Job drawing, mm, ordinate dimensions from the low corner. One solid piece. A direction names the side the tool comes from. Give positions to 0.01 mm unless a question says otherwise; leave off trailing zeros. Order: outer loops, then holes, each group sorted by start corner. A loop starts at its lowest first (then second) coordinate and runs counter-clockwise, first axis right, second up. Notation, with made-up numbers: M -2,43.5 L 35,43.5 A16 cw 35,51.5 Z; hole C 58,-15 d4. An arc over 180 degrees is marked long. Put each result on its own line as item: value. Start each with the question number.
1) Cut at D-D (z = 45). Write the cut outline in (x, y).
2) Cut at A-A (z = 111.4). Write the cut outline in (x, y), and give its area (3 significant figures).
3) Cut at C-C (y = 1.5). Write the cut outline in (x, z), and give its area (3 significant figures).
4) Cut at B-B (x = 44.45). Write the cut outline in (y, z), and give its area (3 significant figures).
5) Pin check, flat tips, straight feed: pin 1 (5.5 mm diameter, centred on y = 3.5, z = 112, fed in from +X); pin 2 (2.5 mm diameter, centred on y = 1.5, z = 110.5, fed in from -X); pin 3 (1.5 mm diameter, centred on x = 62, y = 3, fed in from -Z); pin 4 (4 mm diameter, centred on x = 54.45, z = 7.5, fed in from -Y). Stop position of each tip, or through.
6) Tool access for the marked faces 1 and 2: list every direction of +Z, -Z, +X, -X, +Y, -Y with a clear straight run to the whole face (end or side of a thin tool).
7) Drill centre lines: line 1 (X direction, y = 3.25, z = 111.4); line 2 (Y direction, x = 56, z = 19); line 3 (Z direction, x = 19.5, y = 1.5). Where is each one in solid material? Low to high. Write a range as [from, to].
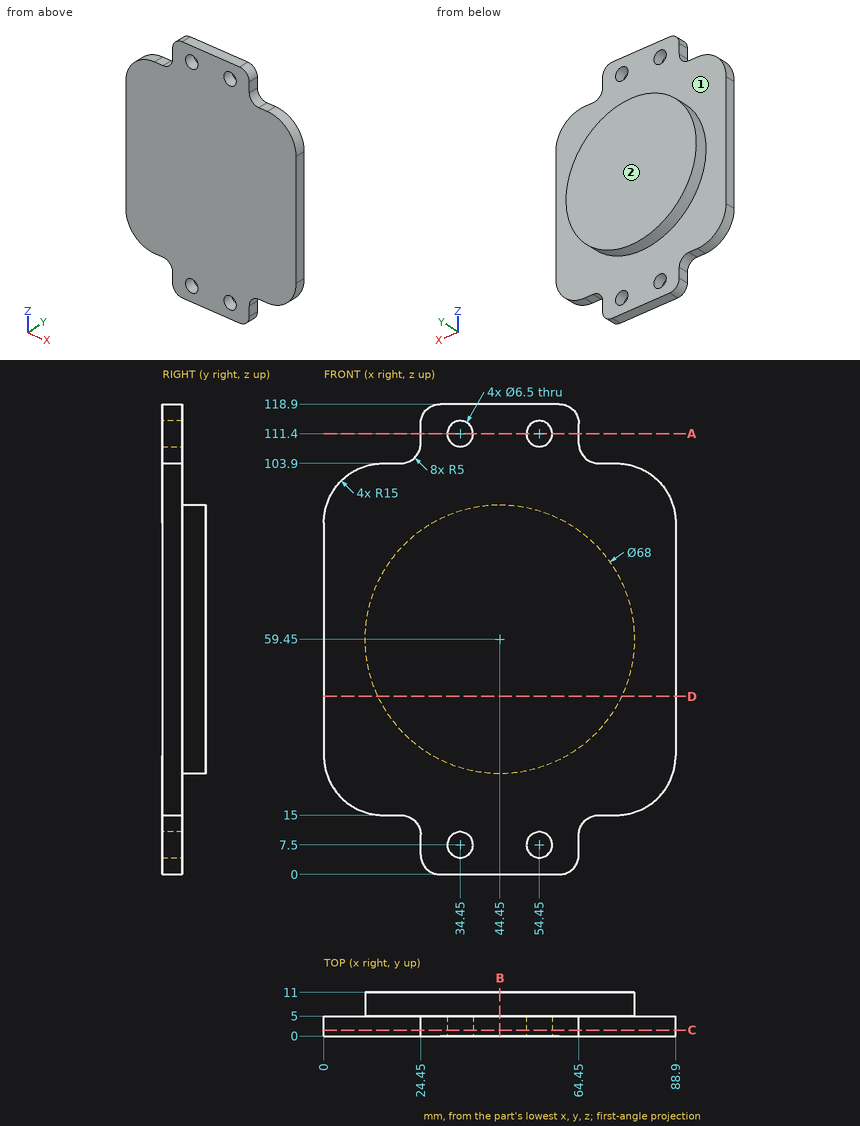
Solution:
1. outline: M 0,0 L 88.9,0 L 88.9,5 L 75.23,5 L 75.23,11 L 13.67,11 L 13.67,5 L 0,5 Z
2. outline: M 24.45,0 L 31.2,0 L 31.2,5 L 24.45,5 Z; M 37.7,0 L 51.2,0 L 51.2,5 L 37.7,5 Z; M 57.7,0 L 64.45,0 L 64.45,5 L 57.7,5 Z
2. area: 135 mm²
3. outline: M 0,30 A15 ccw 15,15 L 19.45,15 A5 cw 24.45,10 L 24.45,5 A5 ccw 29.45,0 L 59.45,0 A5 ccw 64.45,5 L 64.45,10 A5 cw 69.45,15 L 73.9,15 A15 ccw 88.9,30 L 88.9,88.9 A15 ccw 73.9,103.9 L 69.45,103.9 A5 cw 64.45,108.9 L 64.45,113.9 A5 ccw 59.45,118.9 L 29.45,118.9 A5 ccw 24.45,113.9 L 24.45,108.9 A5 cw 19.45,103.9 L 15,103.9 A15 ccw 0,88.9 Z; hole C 34.45,7.5 d6.5; hole C 34.45,111.4 d6.5; hole C 54.45,7.5 d6.5; hole C 54.45,111.4 d6.5
3. area: 8,780 mm²
4. outline: M 0,0 L 5,0 L 5,25.45 L 11,25.45 L 11,93.45 L 5,93.45 L 5,118.9 L 0,118.9 Z
4. area: 1,000 mm²
5. pin 1: x = 64.45
5. pin 2: x = 24.45
5. pin 3: z = 0.34
5. pin 4: through
6. face 1: +Y
6. face 2: +Z, -Z, +X, -X, +Y
7. line 1: [24.45, 31.2], [37.7, 51.2], [57.7, 64.45]
7. line 2: [0, 5]
7. line 3: [15, 103.9]
